The listing builds one solid part. Answer for the finished solid, in the listing's coordinates (mm). A direction names the side the tool comes from. Round coordinates to 2 decimals unless told otherwise and drop trailing zeros. Write each loop counter-clockwise with the first axis right and the second up, starting at its lowest first coordinate (ties: lowest second). Pieces come first, ordered by that corner, then holes. Notation, with made-up numbers: (42, -29.5) -> (66, -29.5) arc R13 cw to (66, -7.5) -> close; hole circle Ø9 at (3, -33). An arc over 180 degrees is marked (long way). Write each question's results on one line, items separated by ' | '. Start each with the question number.
Autodesk Inventor part; units mm, degrees
ref_plane "Work Plane1" through (0, 6, 0) normal (0, 1, 0) x (-1, 0, 0)
ref_plane "YZ Plane" through (0, 0, 0) normal (1, 0, 0) x (0, 1, 0)
ref_plane "XY Plane" through (0, 0, 0) normal (0, 0, 1) x (1, 0, 0)
sketch "Sketch1" plane through (0, 0, 0) normal (0, 0, 1) x (1, 0, 0)
  line L0 (-7, 0) -> (-7, 8)
  line L1 (-7, 8) -> (-5, 8)
  line L2 (-5, 8) -> (-5, 6)
  line L3 (-5, 6) -> (5, 6)
  line L4 (5, 6) -> (5, 8)
  line L5 (5, 8) -> (7, 8)
  line L6 (7, 8) -> (7, 0)
  line L7 (7, 0) -> (-7, 0)
  point P0 (0, 0)
  point P1 (0, 0)
  dimension "d0" = 10
  dimension "d1" = 16
  dimension "d2" = 12
  dimension "d3" = 2
  dimension "d4" = 2
  dimension "d5" = 5
revolve "Revolution1" add sketch "Sketch1" angle 360 about axis through (7, 0, 0) along (-1, 0, 0)
ref_plane "Work Plane1" through (0, 6, 0) normal (0, 1, 0) x (-1, 0, 0)
sketch "Sketch3" plane through (0, 6, 0) normal (0, 1, 0) x (-1, 0, 0)
  point P0 (0, 0)
  point P1 (0, 0)
sketch "Sketch2" plane through (7, 0, 0) normal (1, 0, 0) x (0, 0, -1)
  circle A0 centre (0, 0) radius 8
  point P0 (0, 0)
hole "Hole1" at (7, 0, 0) direction (-1, 0, 0) diameter 8 depth 14
hole "Hole2" at (0, 6, 0) direction (0, -1, 0) diameter 2 end through all
equation "\"d4\" = d3"
properties part number "146" material "Rubber"
Q1. For faces 4 (the cylindrical face through (0, 5, 1)), 5 (the flat face through (5, -2, -6)), determine the directions among +Z, -Z, +X, -X, +Y, -Y from which every point of the face is accessible in a straight line to the end or side of a thin tool.
Q2. Determine the mould class of faces 1 (the cylindrical face through (-5.99, -1.73, -7.81)), 2 (the cylindrical face through (0.07, 5.723, 1.802)), 3 (the flat face through (7, -4, 2)) for opening direction X: pulls with the +X half, pulls with the -X half, needs draft (parallel to the pull), parting line crosses it, or undercut.
Q3. The part is cut by section A-A, the plane z = 0. Write down the section's boundary in (x, y).
Q4. The part is cut by section C-C, the plane x = 0. Write down the section's boundary in (y, z).
Q5. Each of these flat-tipped pins is pushed along its axis until it touches: pin 1 (1.5 mm diameter, centred on x = 3, z = -6, fed in from -Y); pin 2 (4 mm diameter, centred on x = 0, y = -6, fed in from -Z); pin 3 (1 mm diameter, centred on x = -3.5, z = 1.5, fed in from -Y). Where does it stop, or does it pass through?
Q6. The part is cut by section B-B, the plane y = -6.5. Write down the section's boundary in (x, z), then the cut area to 3 significant figures.
Q7. Find the intervals of material crossed by line 1 (X direction, y = 4.75, z = 0); line 2 (X direction, y = -5.5, z = 5.5); line 3 (Z direction, x = 3.75, y = 0), in increasing order.
Q8. The part is cut by section D-D, the plane z = -2. Write down the section's boundary in (x, y).
Answers follow:
1) face 4: +Y, -Y | face 5: none
2) face 1: needs draft | face 2: undercut | face 3: pulls with the +X half
3) outline: (-7, -8) -> (-5, -8) -> (-5, -6) -> (-1, -6) -> (-1, -4) -> (-7, -4) -> close; (-7, 4) -> (-1, 4) -> (-1, 6) -> (-5, 6) -> (-5, 8) -> (-7, 8) -> close; (1, -6) -> (5, -6) -> (5, -8) -> (7, -8) -> (7, -4) -> (1, -4) -> close; (1, 4) -> (7, 4) -> (7, 8) -> (5, 8) -> (5, 6) -> (1, 6) -> close
4) outline: (-5.92, -1) arc R6 ccw to (5.92, -1) -> (3.87, -1) arc R4 cw to (-3.87, -1) -> close; (-5.92, 1) -> (-3.87, 1) arc R4 cw to (3.87, 1) -> (5.92, 1) arc R6 ccw to start
5) pin 1: y = -2.9 | pin 2: z = -4.47 | pin 3: y = -5.92
6) outline: (-7, -4.66) -> (-5, -4.66) -> (-5, 4.66) -> (-7, 4.66) -> close; (5, -4.66) -> (7, -4.66) -> (7, 4.66) -> (5, 4.66) -> close | area: 37.3 mm^2
7) line 1: -7 to -1, 1 to 7 | line 2: -7 to -5, 5 to 7 | line 3: -6 to -4, 4 to 6
8) outline: (-7, -7.75) -> (-5, -7.75) -> (-5, -5.66) -> (5, -5.66) -> (5, -7.75) -> (7, -7.75) -> (7, -3.46) -> (-7, -3.46) -> close; (-7, 3.46) -> (7, 3.46) -> (7, 7.75) -> (5, 7.75) -> (5, 5.66) -> (-5, 5.66) -> (-5, 7.75) -> (-7, 7.75) -> close
